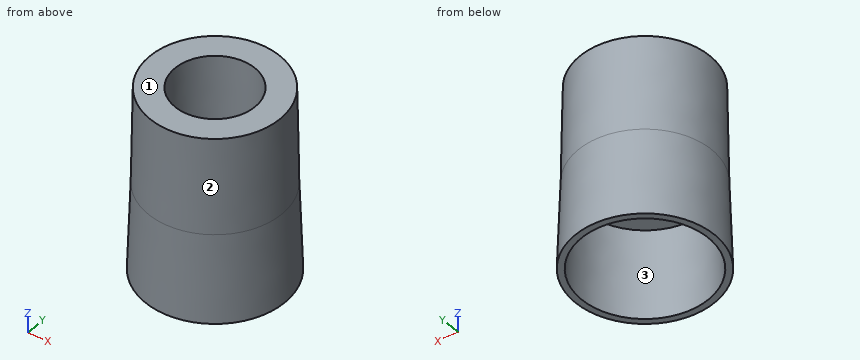
from build123d import *

# Parameters (mm, degrees)
F0_R     = 27.75
F1_DEPTH = 35
F1_TAPER = 2
F2_R     = 25.25
F3_DEPTH = 35.001
F3_TAPER = 1.5
F4_R     = 26.5277730678
F4_R_2   = 15.24
F5_DEPTH = 38.1
F5_TAPER = 1


with BuildPart() as f1:
    # F0 (on Top) → F1 (new body)
    with BuildSketch(Plane.XY):
        Circle(F0_R)
    extrude(amount=F1_DEPTH, taper=F1_TAPER)

    # F2 (on face) → F3 (cut, through all)
    with BuildSketch(Plane(origin=(0, 0, 0), x_dir=(1, 0, 0), z_dir=(0, 0, -1))):
        Circle(F2_R)
    extrude(amount=-F3_DEPTH, taper=F3_TAPER, mode=Mode.SUBTRACT)

    # F4 (on face) → F5 (join)
    with BuildSketch(Plane.XY.offset(35)):
        Circle(F4_R)
        Circle(F4_R_2, mode=Mode.SUBTRACT)
    extrude(amount=F5_DEPTH, taper=F5_TAPER)


solid = f1.part
Can you work these out from the model? Positions are in its coordinate system, mm. Face numbers are marked on the shaded views. Coordinates: 2 decimals unless noted, no trailing zeros. Loops run counter-clockwise (first coordinate to the right, second up) from the corner with the lowest first, then second, coordinate; pieces in that order, holes last. Notation, with made-up numbers: (23.25, 53) - (75.25, 53) arc R30 ccw to (75.25, 91) - close; hole circle Ø7 at (84, -5.75). An arc over 180 degrees is marked (long way). Put each result on its own line as item: value. Start each with the question number.
Item 1: If we mould it in two halves opening along X, with no side actions, what happens to the marked faces 1, 2 and 3? For each: +X half, -X half, draft (parallel to the pull), parting line (faces both ways), or undercut.
Item 2: For pin 1 (1 mm diameter, centred on y = 6.5, z = 40.5, fed in from +X); pin 2 (5 mm diameter, centred on y = -12.5, z = 35.5, fed in from -X); pin 3 (12 mm diameter, centred on x = -13.5, z = 46, fed in from +Y), each with a flat end and sliding along its axis, tell me the tip position at first contact or that it passes through.
Item 3: Suppose I cut it at A-A (z = 64). Please give me the cut outline in (x, y), and give its area (3 significant figures).
Item 4: Suppose I cut it at B-B (z = 29.5). Please give me the cut outline in (x, y), and give its area (3 significant figures).
Item 5: If I drill on line 1 along Z through (x, y) = (16, 12); line 2 along X through (y, z) = (-1, 46); line 3 along Y through (x, z) = (3.5, 15.5), over which ranges is the centre line in solid material (lowest first)?
Here are the results:
1. face 1: draft
1. face 2: parting line
1. face 3: undercut
2. pin 1: x = 25.74
2. pin 2: x = -24.56
2. pin 3: y = 25.25
3. outline: circle Ø52.04 at (0, 0); hole circle Ø31.49 at (0, 0)
3. area: 1,350 mm²
4. outline: circle Ø53.44 at (0, 0); hole circle Ø48.96 at (0, 0)
4. area: 361 mm²
5. line 1: 35 to 73.1
5. line 2: -26.32 to -15.4, 15.4 to 26.32
5. line 3: -26.98 to -24.6, 24.6 to 26.98
